Source: CAD feature listing. Evaluate the final solid. Frame: model axes, mm. A direction names the side the tool comes from. Coordinates: 2 decimals unless noted, no trailing zeros. Write each loop counter-clockwise with the first axis right and the second up, starting at its lowest first coordinate (ties: lowest second). Pieces come first, ordered by that corner, then holes. Notation, with made-up numbers: (-40, 15) -> (2, 15) arc R33 cw to (2, 51) -> close; hole circle Ø10 at (21, 46). An arc over 180 degrees is marked (long way). One line per item, written item: value. Start each with the question number.
1. Access query for faces 1 (the flat face through (-18, 33.635, 0)), 2 (the flat face through (-61.89, 16, 0)), 3 (the flat face through (-40.158, 40, 0)), 4 (the flat face through (-42, 16, 10)), 5 (the flat face through (-28.683, 40, 0)). Directions: +Z, -Z, +X, -X, +Y, -Y. A direction counts if a zero-diameter tool reaches every point of the face in a straight line with its end or side. Return the directions, or none.
2. Section query C-C, the plane y = 39. Output: boundary loops of the cut face in (x, z), and give its area (3 significant figures).
3. First-contact query: P1, Ø6, axis at x = -64, z = -1, coming from the -Y side; P2, Ø6, axis at x = -18, z = -1, coming from the -Y side; P3, Ø4, axis at x = -19.5, z = 2, coming from the +Y side; P4, Ø3, axis at y = 3.5, z = 2.5, coming from the +X side. Flat tips, straight axial feed; report the tip coordinate or a pass-through.
4. Line query: line 1 (X direction, y = 7, z = 7.75); line 2 (Y direction, x = -50, z = -5.5); line 3 (Y direction, x = -62, z = -8.75). Output: solid intervals per line, ascending.
5. Section query B-B, the plane x = -53. Output: boundary loops of the cut face in (y, z), and give its area (3 significant figures).
6. Section query A-A, the plane z = 4.5. Output: boundary loops of the cut face in (x, y).
Autodesk Inventor part; units mm, degrees
ref_plane "YZ Plane" through (0, 0, 0) normal (1, 0, 0) x (0, 1, 0)
ref_plane "XZ Plane" through (0, 0, 0) normal (0, 1, 0) x (-1, 0, 0)
ref_plane "XY Plane" through (0, 0, 0) normal (0, 0, 1) x (1, 0, 0)
sketch "Sketch1" plane through (0, 0, 0) normal (0, 0, 1) x (1, 0, 0)
  line L0 (-69.1405, 36.1754) -> (-69.1405, 33.6354)
  line L1 (-69.1405, 33.6354) -> (-61.8905, 33.6354)
  line L2 (-61.8905, 33.6354) -> (-61.8905, -2.9246)
  line L3 (-61.8905, -2.9246) -> (-21.8905, -2.9246)
  line L4 (-21.8905, -2.9246) -> (-21.8905, 33.6354)
  line L5 (-21.8905, 33.6354) -> (-14.6405, 33.6354)
  line L6 (-14.6405, 33.6354) -> (-14.6405, 36.1754)
  line L7 (-14.6405, 36.1754) -> (-21.8905, 36.1754)
  line L8 (-21.8905, 36.1754) -> (-21.8905, 36.1754)
  line L9 (-21.8905, 36.1754) -> (-28.6829, 36.1754)
  line L10 (-28.6829, 36.1754) -> (-28.6829, 44.1754)
  line L11 (-28.6829, 44.1754) -> (-40.1582, 44.1754)
  line L12 (-40.1582, 44.1754) -> (-40.1582, 36.1754)
  line L13 (-40.1582, 36.1754) -> (-61.8905, 36.1754)
  line L14 (-61.8905, 36.1754) -> (-61.8905, 36.1754)
  line L15 (-61.8905, 36.1754) -> (-69.1405, 36.1754)
  dimension "d7" = 47.1
  dimension "d8" = 40
  dimension "d9" = 39.1
  dimension "d10" = 54.5
  dimension "d11" = 39.1
  dimension "d12" = 2.54
extrude "Extrusion1" add sketch "Sketch1" along normal mid plane 20
properties part number "FUTABA-RS404PD Blank"
Computed values:
1. face 1: +Z, -Z, +X, -Y
1. face 2: +Z, -Z, -X, -Y
1. face 3: +Z, -Z, -X, +Y
1. face 4: +Z, +X, -X, +Y, -Y
1. face 5: +Z, -Z, +X, +Y
2. outline: (-40.16, -10) -> (-28.68, -10) -> (-28.68, 10) -> (-40.16, 10) -> close
2. area: 230 mm²
3. P1: stops at y = -2.92
3. P2: stops at y = 33.64
3. P3: stops at y = 36.18
3. P4: stops at x = -21.89
4. line 1: x = -61.89 to -21.89
4. line 2: y = -2.92 to 36.18
4. line 3: y = 33.64 to 36.18
5. outline: (-2.92, -10) -> (36.18, -10) -> (36.18, 10) -> (-2.92, 10) -> close
5. area: 782 mm²
6. outline: (-69.14, 33.64) -> (-61.89, 33.64) -> (-61.89, -2.92) -> (-21.89, -2.92) -> (-21.89, 33.64) -> (-14.64, 33.64) -> (-14.64, 36.18) -> (-28.68, 36.18) -> (-28.68, 44.18) -> (-40.16, 44.18) -> (-40.16, 36.18) -> (-69.14, 36.18) -> close
